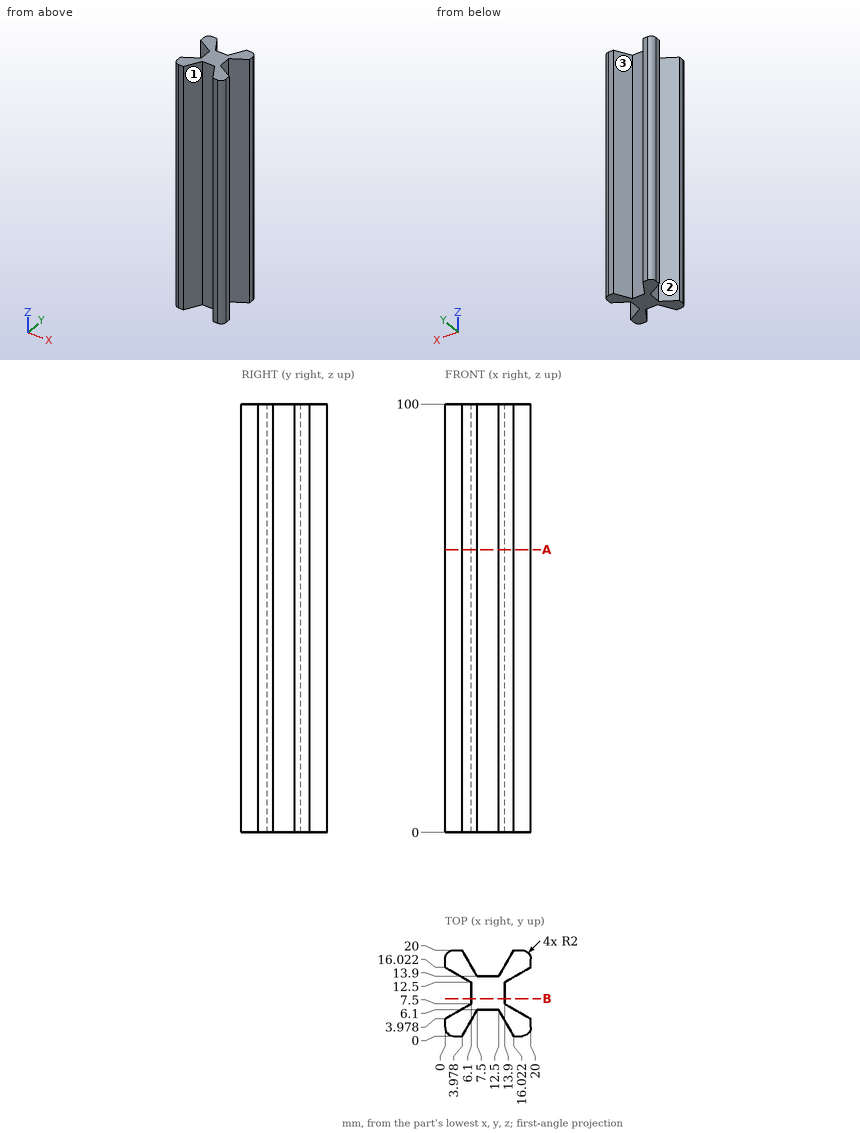
The drawing under review shows one solid part. Ordinate dimensions are in mm from its lowest x, y, z. Give positions to 0.01 mm unless a question says otherwise; leave off trailing zeros. Write each loop counter-clockwise with the first axis right and the second up, starting at its lowest first coordinate (ties: lowest second). Pieces come first, ordered by that corner, then holes. Notation, with made-up numbers: (7.25, 55) -> (11.25, 55) arc R34 cw to (11.25, 87) -> close; hole circle Ø11 at (72.5, 40). An arc over 180 degrees is marked (long way). Put each result on its own line as item: value.
(1) We need section B-B, the plane y = 8.75. Give the boundary of the cut face in (x, z), and give its area (3 significant figures).
Results are:
outline: (6.1, 0) -> (13.9, 0) -> (13.9, 100) -> (6.1, 100) -> close
area: 780 mm²
(2) To check wall thickness, follow probe 1 along X at (y, z) = (12.5, 31.5); probe 2 along X at (y, z) = (5.75, 89.5); probe 3 along Y at (x, z) = (3.5, 85). State the ranges of each line that lie inside material, in increasing order. Write a range as from..to.
Results are:
probe 1: 6.1..13.9
probe 2: 3.07..7.3, 12.7..16.93
probe 3: 0..6, 14..20
(3) The part is to be moulded in two halves that separate along Y. For the marked faces 1, 2 and 3, say which applies: pulls with the +Y half, pulls with the -Y half, needs draft (parallel to the pull), parting line crosses it, or undercut.
Results are:
face 1: pulls with the -Y half
face 2: undercut
face 3: pulls with the +Y half
(4) We need section A-A, the plane z = 66. Give the boundary of the cut face in (x, y).
Results are:
outline: (0, 2) arc R2 ccw to (2, 0) -> (3.98, 0) -> (7.5, 6.1) -> (12.5, 6.1) -> (16.02, 0) -> (18, 0) arc R2 ccw to (20, 2) -> (20, 3.98) -> (13.9, 7.5) -> (13.9, 12.5) -> (20, 16.02) -> (20, 18) arc R2 ccw to (18, 20) -> (16.02, 20) -> (12.5, 13.9) -> (7.5, 13.9) -> (3.98, 20) -> (2, 20) arc R2 ccw to (0, 18) -> (0, 16.02) -> (6.1, 12.5) -> (6.1, 7.5) -> (0, 3.98) -> close
(5) For pin 1 Ø1.5 at (x, z) = (13, 21) entering from -Y (1 decimal); pin 2 Ø12 at (y, z) = (7, 86) entering from -X; pin 3 Ø1 at (x, z) = (15, 33.5) entering from +Y; pin 4 Ø5.5 at (y, z) = (10.5, 33.5) entering from +X, all flat-tipped, find the tip position at first contact; note any pin that passes through.
Results are:
pin 1: y = 3.9
pin 2: x = 0
pin 3: y = 19.1
pin 4: x = 15.2
